Geometry: final body of the model. Coordinates: model frame, mm. A direction names the side the tool comes from. Round coordinates to 2 decimals unless told otherwise and drop trailing zeros. Write each loop counter-clockwise with the first axis right and the second up, starting at its lowest first coordinate (ties: lowest second). Pieces come first, ordered by that corner, then holes. Notation, with made-up numbers: M 77,71 L 128,71 A15 ccw 128,86 Z; hole C -22.75,37 d2. An arc over 180 degrees is marked long. Use one line per item in the form item = value. Start each with the question number.
Item 1: Ray query, probe 1 along X at (y, z) = (-15, 0.75); probe 2 along X at (y, z) = (-22, 5); probe 3 along Y at (x, z) = (-7, 3). Return the intervals inside material, ascending.
Item 2: Section query B-B (x = -13.5). Return loops of the section in (y, z), and give its area (3 significant figures).
Item 3: Pin query (flat end, axial travel): pin 1 Ø2 at (x, z) = (-16, 1.5) entering from -Y; pin 2 Ø5 at (x, y) = (6.91, -6.91) entering from +Z; pin 3 Ø1.5 at (x, z) = (17, 2) entering from +Y; pin 4 Ø2 at (x, y) = (-6.91, 6.91) entering from -Z. Return the tip coordinate at first contact, or that it passes through.
Item 4: Reachability of faces 1 (the cylindrical face through (26.128, -8.578, 3.131)), 2 (the cylindrical face through (-21.617, -3.346, 3.131)), 3 (the cylindrical face through (5.964, 24.127, 3.131)), 4 (the cylindrical face through (24.127, -5.964, 3.131)), 5 (the cylindrical face through (9.356, -23.025, 3.131)) from +Z, -Z, +X, -X, +Y, -Y: full face, straight path, thin tool, end or side. Return the list, or none.
Item 5: Pull-direction query (X, two-part tool) for faces 6 (the cylindrical face through (9.478, 22.89, 3.131)), 7 (the cylindrical face through (24.089, 5.786, 3.131)), 8 (the cylindrical face through (-21, 13, 3)); classes: pulls with the +X half, pulls with the -X half, needs draft (parallel to the pull), parting line crosses it, or undercut.
Item 6: Section query D-D (x = 18). Return loops of the section in (y, z), and give its area (3 significant figures).
Item 7: Section query A-A (y = 6). Return loops of the section in (x, z), and give its area (3 significant figures).
Item 8: Section query C-C (z = 5). State how many separate pieces and enclosed holes the cut face has, and give its area (3 significant figures).
from build123d import *

# Parameters (mm, degrees)
BOSS_EXTRU_1_DEPTH      = 6.35
ENL_V_MAT_EXTRU_1_REACH = 41.406
ESQUISSE2_R             = 3.15
ESQUISSE2_R_2           = 1.83


with BuildPart() as part:
    # Esquisse1 → Boss.-Extru.1 (new body)
    with BuildSketch(Plane.XY):
        with BuildLine():
            ThreePointArc((4.580283008, -21.38908328), (5.809239787, -24.124430095), (7.79392735, -26.37242303))
            ThreePointArc((7.79392735, -26.37242303), (8.426297829, -26.177232568), (9.053788111, -25.96688123))
            ThreePointArc((9.053788111, -25.96688123), (9.354446156, -22.983248931), (8.756985681, -20.044627155))
            ThreePointArc((8.756985681, -20.044627155), (9.877166912, -19.517004119), (10.965698229, -18.926841743))
            ThreePointArc((10.965698229, -18.926841743), (12.979774233, -21.148542625), (15.561992292, -22.673208769))
            ThreePointArc((15.561992292, -22.673208769), (16.103095187, -22.292158383), (16.634871772, -21.898197212))
            ThreePointArc((16.634871772, -21.898197212), (15.998821478, -18.967685826), (14.522518732, -16.357515878))
            ThreePointArc((14.522518732, -16.357515878), (15.424829906, -15.509561514), (16.277714505, -14.611909064))
            ThreePointArc((16.277714505, -14.611909064), (18.879757941, -16.102488453), (21.806741003, -16.75458286))
            ThreePointArc((21.806741003, -16.75458286), (22.203609392, -16.224972418), (22.587618281, -15.685965077))
            ThreePointArc((22.587618281, -15.685965077), (21.077120684, -13.095433477), (18.866486465, -11.069216977))
            ThreePointArc((18.866486465, -11.069216977), (19.462603078, -9.983934966), (19.996354671, -8.86666092))
            ThreePointArc((19.996354671, -8.86666092), (22.9316594, -9.480210518), (25.916893968, -9.195901645))
            ThreePointArc((25.916893968, -9.195901645), (26.130679608, -8.569573106), (26.329331336, -7.93828139))
            ThreePointArc((26.329331336, -7.93828139), (24.092244465, -5.941308858), (21.363671052, -4.697385994))
            ThreePointArc((21.363671052, -4.697385994), (21.595241057, -3.481011302), (21.75761232, -2.253482226))
            ThreePointArc((21.75761232, -2.253482226), (24.738850262, -1.929943525), (27.490120777, -0.737061506))
            ThreePointArc((27.490120777, -0.737061506), (27.499896841, -0.075324271), (27.493745992, 0.586456589))
            ThreePointArc((27.493745992, 0.586456589), (24.749051496, 1.794392467), (21.769630667, 2.134257858))
            ThreePointArc((21.769630667, 2.134257858), (21.613986378, 3.362658002), (21.38908328, 4.580283008))
            ThreePointArc((21.38908328, 4.580283008), (24.124430095, 5.809239787), (26.37242303, 7.79392735))
            ThreePointArc((26.37242303, 7.79392735), (26.177232568, 8.426297829), (25.96688123, 9.053788111))
            ThreePointArc((25.96688123, 9.053788111), (22.983248931, 9.354446156), (20.044627155, 8.756985681))
            ThreePointArc((20.044627155, 8.756985681), (19.517004119, 9.877166912), (18.926841743, 10.965698229))
            ThreePointArc((18.926841743, 10.965698229), (21.148542625, 12.979774233), (22.673208769, 15.561992292))
            ThreePointArc((22.673208769, 15.561992292), (22.292158383, 16.103095187), (21.898197212, 16.634871772))
            ThreePointArc((21.898197212, 16.634871772), (18.967685826, 15.998821478), (16.357515878, 14.522518732))
            ThreePointArc((16.357515878, 14.522518732), (15.509561514, 15.424829906), (14.611909064, 16.277714505))
            ThreePointArc((14.611909064, 16.277714505), (16.102488453, 18.879757941), (16.75458286, 21.806741003))
            ThreePointArc((16.75458286, 21.806741003), (16.224972418, 22.203609392), (15.685965077, 22.587618281))
            ThreePointArc((15.685965077, 22.587618281), (13.095433477, 21.077120684), (11.069216977, 18.866486465))
            ThreePointArc((11.069216977, 18.866486465), (9.983934966, 19.462603078), (8.86666092, 19.996354671))
            ThreePointArc((8.86666092, 19.996354671), (9.480210518, 22.9316594), (9.195901645, 25.916893968))
            ThreePointArc((9.195901645, 25.916893968), (8.569573106, 26.130679608), (7.93828139, 26.329331336))
            ThreePointArc((7.93828139, 26.329331336), (5.941308858, 24.092244465), (4.697385994, 21.363671052))
            ThreePointArc((4.697385994, 21.363671052), (3.481011302, 21.595241057), (2.253482226, 21.75761232))
            ThreePointArc((2.253482226, 21.75761232), (1.929943525, 24.738850262), (0.737061506, 27.490120777))
            ThreePointArc((0.737061506, 27.490120777), (0.075324271, 27.499896841), (-0.586456589, 27.493745992))
            ThreePointArc((-0.586456589, 27.493745992), (-1.794392467, 24.749051496), (-2.134257858, 21.769630667))
            ThreePointArc((-2.134257858, 21.769630667), (-3.362658002, 21.613986378), (-4.580283008, 21.38908328))
            ThreePointArc((-4.580283008, 21.38908328), (-5.809239787, 24.124430095), (-7.79392735, 26.37242303))
            ThreePointArc((-7.79392735, 26.37242303), (-8.426297829, 26.177232568), (-9.053788111, 25.96688123))
            ThreePointArc((-9.053788111, 25.96688123), (-9.354446156, 22.983248931), (-8.756985681, 20.044627155))
            ThreePointArc((-8.756985681, 20.044627155), (-9.877166912, 19.517004119), (-10.965698229, 18.926841743))
            ThreePointArc((-10.965698229, 18.926841743), (-12.979774233, 21.148542625), (-15.561992292, 22.673208769))
            ThreePointArc((-15.561992292, 22.673208769), (-16.103095187, 22.292158383), (-16.634871772, 21.898197212))
            ThreePointArc((-16.634871772, 21.898197212), (-15.998821478, 18.967685826), (-14.522518732, 16.357515878))
            ThreePointArc((-14.522518732, 16.357515878), (-15.424829906, 15.509561514), (-16.277714505, 14.611909064))
            ThreePointArc((-16.277714505, 14.611909064), (-18.879757941, 16.102488453), (-21.806741003, 16.75458286))
            ThreePointArc((-21.806741003, 16.75458286), (-22.203609392, 16.224972418), (-22.587618281, 15.685965077))
            ThreePointArc((-22.587618281, 15.685965077), (-21.077120684, 13.095433477), (-18.866486465, 11.069216977))
            ThreePointArc((-18.866486465, 11.069216977), (-19.462603078, 9.983934966), (-19.996354671, 8.86666092))
            ThreePointArc((-19.996354671, 8.86666092), (-22.9316594, 9.480210518), (-25.916893968, 9.195901645))
            ThreePointArc((-25.916893968, 9.195901645), (-26.130679608, 8.569573106), (-26.329331336, 7.93828139))
            ThreePointArc((-26.329331336, 7.93828139), (-24.092244465, 5.941308858), (-21.363671052, 4.697385994))
            ThreePointArc((-21.363671052, 4.697385994), (-21.595241057, 3.481011302), (-21.75761232, 2.253482226))
            ThreePointArc((-21.75761232, 2.253482226), (-24.738850262, 1.929943525), (-27.490120777, 0.737061506))
            ThreePointArc((-27.490120777, 0.737061506), (-27.499896841, 0.075324271), (-27.493745992, -0.586456589))
            ThreePointArc((-27.493745992, -0.586456589), (-24.749051496, -1.794392467), (-21.769630667, -2.134257858))
            ThreePointArc((-21.769630667, -2.134257858), (-21.613986378, -3.362658002), (-21.38908328, -4.580283008))
            ThreePointArc((-21.38908328, -4.580283008), (-24.124430095, -5.809239787), (-26.37242303, -7.79392735))
            ThreePointArc((-26.37242303, -7.79392735), (-26.177232568, -8.426297829), (-25.96688123, -9.053788111))
            ThreePointArc((-25.96688123, -9.053788111), (-22.983248931, -9.354446156), (-20.044627155, -8.756985681))
            ThreePointArc((-20.044627155, -8.756985681), (-19.517004119, -9.877166912), (-18.926841743, -10.965698229))
            ThreePointArc((-18.926841743, -10.965698229), (-21.148542625, -12.979774233), (-22.673208769, -15.561992292))
            ThreePointArc((-22.673208769, -15.561992292), (-22.292158383, -16.103095187), (-21.898197212, -16.634871772))
            ThreePointArc((-21.898197212, -16.634871772), (-18.967685826, -15.998821478), (-16.357515878, -14.522518732))
            ThreePointArc((-16.357515878, -14.522518732), (-15.509561514, -15.424829906), (-14.611909064, -16.277714505))
            ThreePointArc((-14.611909064, -16.277714505), (-16.102488453, -18.879757941), (-16.75458286, -21.806741003))
            ThreePointArc((-16.75458286, -21.806741003), (-16.224972418, -22.203609392), (-15.685965077, -22.587618281))
            ThreePointArc((-15.685965077, -22.587618281), (-13.095433477, -21.077120684), (-11.069216977, -18.866486465))
            ThreePointArc((-11.069216977, -18.866486465), (-9.983934966, -19.462603078), (-8.86666092, -19.996354671))
            ThreePointArc((-8.86666092, -19.996354671), (-9.480210518, -22.9316594), (-9.195901645, -25.916893968))
            ThreePointArc((-9.195901645, -25.916893968), (-8.569573106, -26.130679608), (-7.93828139, -26.329331336))
            ThreePointArc((-7.93828139, -26.329331336), (-5.941308858, -24.092244465), (-4.697385994, -21.363671052))
            ThreePointArc((-4.697385994, -21.363671052), (-3.481011302, -21.595241057), (-2.253482226, -21.75761232))
            ThreePointArc((-2.253482226, -21.75761232), (-1.929943525, -24.738850262), (-0.737061506, -27.490120777))
            ThreePointArc((-0.737061506, -27.490120777), (-0.075324271, -27.499896841), (0.586456589, -27.493745992))
            ThreePointArc((0.586456589, -27.493745992), (1.794392467, -24.749051496), (2.134257858, -21.769630667))
            ThreePointArc((2.134257858, -21.769630667), (3.362658002, -21.613986378), (4.580283008, -21.38908328))
        make_face()
    extrude(amount=BOSS_EXTRU_1_DEPTH)

    # Esquisse2 → Enlèv. mat.-Extru.1 (cut, up to next)
    with BuildSketch(Plane(origin=(0, 0, 0), x_dir=(-1, 0, 0), z_dir=(0, 0, -1)), mode=Mode.PRIVATE) as enl_v_mat_extru_1_sk1:
        Circle(ESQUISSE2_R)
    enl_v_mat_extru_1_tool1 = extrude(enl_v_mat_extru_1_sk1.sketch, amount=-ENL_V_MAT_EXTRU_1_REACH, mode=Mode.PRIVATE) & part.part
    # Esquisse2 → Enlèv. mat.-Extru.1 (cut, up to next)
    with BuildSketch(Plane(origin=(0, 0, 0), x_dir=(-1, 0, 0), z_dir=(0, 0, -1)), mode=Mode.PRIVATE) as enl_v_mat_extru_1_sk2:
        with Locations((-6.914797213, -6.914797213)):
            Circle(ESQUISSE2_R_2)
    enl_v_mat_extru_1_tool2 = extrude(enl_v_mat_extru_1_sk2.sketch, amount=-ENL_V_MAT_EXTRU_1_REACH, mode=Mode.PRIVATE) & part.part
    # Esquisse2 → Enlèv. mat.-Extru.1 (cut, up to next)
    with BuildSketch(Plane(origin=(0, 0, 0), x_dir=(-1, 0, 0), z_dir=(0, 0, -1)), mode=Mode.PRIVATE) as enl_v_mat_extru_1_sk3:
        with Locations((-6.914797213, 6.914797213)):
            Circle(ESQUISSE2_R_2)
    enl_v_mat_extru_1_tool3 = extrude(enl_v_mat_extru_1_sk3.sketch, amount=-ENL_V_MAT_EXTRU_1_REACH, mode=Mode.PRIVATE) & part.part
    # Esquisse2 → Enlèv. mat.-Extru.1 (cut, up to next)
    with BuildSketch(Plane(origin=(0, 0, 0), x_dir=(-1, 0, 0), z_dir=(0, 0, -1)), mode=Mode.PRIVATE) as enl_v_mat_extru_1_sk4:
        with Locations((6.914797213, 6.914797213)):
            Circle(ESQUISSE2_R_2)
    enl_v_mat_extru_1_tool4 = extrude(enl_v_mat_extru_1_sk4.sketch, amount=-ENL_V_MAT_EXTRU_1_REACH, mode=Mode.PRIVATE) & part.part
    # Esquisse2 → Enlèv. mat.-Extru.1 (cut, up to next)
    with BuildSketch(Plane(origin=(0, 0, 0), x_dir=(-1, 0, 0), z_dir=(0, 0, -1)), mode=Mode.PRIVATE) as enl_v_mat_extru_1_sk5:
        with Locations((6.914797213, -6.914797213)):
            Circle(ESQUISSE2_R_2)
    enl_v_mat_extru_1_tool5 = extrude(enl_v_mat_extru_1_sk5.sketch, amount=-ENL_V_MAT_EXTRU_1_REACH, mode=Mode.PRIVATE) & part.part
    add(enl_v_mat_extru_1_tool1.solids().sort_by_distance((0, 0, 0))[0], mode=Mode.SUBTRACT)
    add(enl_v_mat_extru_1_tool2.solids().sort_by_distance((6.914797, -6.914797, 0))[0], mode=Mode.SUBTRACT)
    add(enl_v_mat_extru_1_tool3.solids().sort_by_distance((6.914797, 6.914797, 0))[0], mode=Mode.SUBTRACT)
    add(enl_v_mat_extru_1_tool4.solids().sort_by_distance((-6.914797, 6.914797, 0))[0], mode=Mode.SUBTRACT)
    add(enl_v_mat_extru_1_tool5.solids().sort_by_distance((-6.914797, -6.914797, 0))[0], mode=Mode.SUBTRACT)


solid = part.part
Working result:
q1.probe_1 = -22.43 to -17.02, -15.92 to 15.92, 16.8 to 22.29
q1.probe_2 = -16.5 to -14.46, -9.38 to -4.9, -2.26 to 2.14, 4.77 to 9.26, 14.2 to 16.5
q1.probe_3 = -25.44 to -8.74, -5.09 to 5.09, 8.74 to 25.63
q2.outline = M -21.39,0 L 21.54,0 L 21.54,6.35 L -21.39,6.35 Z
q2.area = 273 mm²
q3.pin_1 = -22.59
q3.pin_2 = 6.35
q3.pin_3 = 22.19
q3.pin_4 = through
q4.face_1 = +Z, -Z, +X, -Y
q4.face_2 = +Z, -Z, -X
q4.face_3 = +Z, -Z, +Y
q4.face_4 = +Z, -Z, +X
q4.face_5 = +Z, -Z
q5.face_6 = undercut
q5.face_7 = pulls with the +X half
q5.face_8 = pulls with the -X half
q6.outline = M -15.71,0 L 15.57,0 L 15.57,6.35 L -15.71,6.35 Z
q6.area = 199 mm²
q7.outline = M -24.18,0 L -8.5,0 L -8.5,6.35 L -24.18,6.35 Z; M -5.33,0 L 5.33,0 L 5.33,6.35 L -5.33,6.35 Z; M 8.5,0 L 24.41,0 L 24.41,6.35 L 8.5,6.35 Z
q7.area = 268 mm²
q8.separate_pieces = 1
q8.enclosed_holes = 5
q8.area = 1,820 mm²
